Check sheet for the modelled part. Datum: model origin and axes. Units: mm. A direction names the side the tool comes from. Round coordinates to 2 decimals unless told otherwise and drop trailing zeros. Order: outer loops, then holes, each group sorted by start corner. A loop starts at its lowest first (then second) coordinate and runs counter-clockwise, first axis right, second up.
Autodesk Inventor part; units mm, degrees
ref_plane "YZ Plane" through (0, 0, 0) normal (1, 0, 0) x (0, 1, 0)
ref_plane "XZ Plane" through (0, 0, 0) normal (0, 1, 0) x (-1, 0, 0)
ref_plane "XY Plane" through (0, 0, 0) normal (0, 0, 1) x (1, 0, 0)
sketch "Sketch1" plane through (0, 0, 0) normal (0, 0, 1) x (1, 0, 0)
  line L0 (-16.7671, 64.9713) -> (-16.7671, -55.0287)
  line L1 (-16.7671, -55.0287) -> (11.7813, -55.0287)
  line L2 (11.7813, -55.0287) -> (33.2329, -37.0287)
  line L3 (33.2329, -37.0287) -> (33.2329, -21.0287)
  line L4 (33.2329, -21.0287) -> (-16.7671, 64.9713)
  line L5 (-1.7671, -43.0287) -> (-11.7671, -43.0287)
  line L6 (-11.7671, -43.0287) -> (-11.7671, -45.0287)
  line L7 (-11.7671, -45.0287) -> (-1.7671, -45.0287)
  line L8 (-1.7671, -45.0287) -> (-1.7671, -43.0287)
  line L9 (-16.7671, -40.0287) -> (-18.7671, -40.0287)
  line L10 (-18.7671, -40.0287) -> (-18.7671, -10.0287)
  line L11 (-18.7671, -10.0287) -> (-16.7671, -10.0287)
  line L12 (-16.7671, -10.0287) -> (-16.7671, -40.0287)
  line L13 (-16.7671, 9.9713) -> (-18.7671, 9.9713)
  line L14 (-18.7671, 9.9713) -> (-18.7671, 39.9713)
  line L15 (-18.7671, 39.9713) -> (-16.7671, 39.9713)
  line L16 (-16.7671, 39.9713) -> (-16.7671, 9.9713)
  line L17 (-16.7671, 54.9713) -> (-10.9532, 54.9713)
  circle A0 centre (19.2329, -29.0287) radius 9.5
  line L18 (19.2329, -29.0287) -> (33.2329, -29.0287)
  point P0 (0, 0)
  point P1 (-17.7671, -40.0287)
  point P2 (-17.7671, -10.0287)
  dimension "d0" = 120
  dimension "d1" = 10
  dimension "d2" = 2
  dimension "d3" = 10
  dimension "d4" = 5
  dimension "d5" = 2
  dimension "d6" = 30
  dimension "d7" = 15
  dimension "d8" = 2
  dimension "d9" = 30
  dimension "d10" = 20
  dimension "d11" = 18
  dimension "d12" = 16
  dimension "d13" = 50
  dimension "d14" = 10
  dimension "d15" = 50
  dimension "d16" = 19
  dimension "d17" = 36
  dimension "d18" = 90
extrude "Plate1" add sketch "Sketch1" along normal blind 3 contours L17 L4 L3 L2 L1 L0 | L0 L13 L14 L15 | L0 L9 L10 L11
chamfer "Corner Chamfer1" distance 15 angle 45 1 edges at (11.7813, -55.0287, 1.5)
fillet "Corner Round1" radius 17 4 edges at (33.2329, -37.0287, 1.5) (33.2329, -21.0287, 1.5) (23.272, -45.3869, 1.5) (-3.2187, -55.0287, 1.5)
equation "\"d2\" = d19"
equation "\"d5\" = d19"
equation "\"d8\" = d19"
equation "\"d21\" = Thickness"
equation "\"Thickness\" = plate_thickness"
equation "\"BendRadius\" = Thickness"
equation "\"BendReliefWidth\" = Thickness"
equation "\"BendReliefDepth\" = 0.5 * Thickness"
equation "\"CornerReliefSize\" = 4 * Thickness"
equation "\"MinimumRemnant\" = 2 * Thickness"
equation "\"TransitionRadius\" = BendRadius"
equation "\"JacobiRadiusSize\" = BendRadius"
equation "\"GapSize\" = Thickness"
equation "\"A_width\" = 46"
equation "\"A_joint_diameter\" = 16"
equation "\"A_joint_tolerance\" = 3"
equation "\"l___________\" = 0"
equation "\"l__________\" = 0"
equation "\"l_________\" = 0"
equation "\"rivet_diameter\" = 3.35"
equation "\"plate_thickness\" = 3"
equation "\"l________\" = 0"
equation "\"L_Piston_Top\" = 25"
equation "\"L_Piston_Bottom\" = 21"
equation "\"A_B_spacing\" = 2"
equation "\"thin_plate\" = 1.5"
properties part number "Piston_FloorHinge01" material "Stainless Steel"
1) Set-up check for faces 5 (the face through (-12, -55.029, 1)), 6 (the face through (-11.767, -44, 1)), 7 (the face through (-18, -40.029, 1)), 8 (the face through (-16.767, 0, 1)), 9 (the face through (-16.767, 48, 1)): record each of +Z, -Z, +X, -X, +Y, -Y from which the full face is reachable in a straight line by a thin tool's end or side.
2) Sectioned sample at D-D on x = 5.5. Record the cut outline in (y, z), and give its area (3 significant figures).
3) Draft check along Y on faces 1 (the face through (1, -11, 3)), 2 (the face through (-3.31, -54.78, 1.52)), 3 (the face through (-18, 39.971, 1)), 4 (the face through (-18, -10.029, 1)). Enter one of: pulls with the +Y half, pulls with the -Y half, needs draft (parallel to the pull), parting line crosses it, or undercut.
4) Gauge pin test, flat ends, axial feed: pin 1 (0.6 mm diameter, centred on y = -44, z = 2, fed in from -X); pin 2 (1 mm diameter, centred on x = -17.5, z = 1, fed in from +Y); pin 3 (1 mm diameter, centred on x = -18, z = 2, fed in from -Y). Record the tip position at first contact, or that the pin passes through.
5) Sectioned sample at B-B on z = 1.3. Record the cut outline in (x, y), and give its area (3 significant figures).
6) Sectioned sample at A-A on x = 22. Record the cut outline in (y, z), and give its area (3 significant figures).
7) Scan lines: line 1 (Y direction, x = -8, z = 0.8); line 2 (Y direction, x = 17, z = 2.6); line 3 (X direction, y = -23, z = 0.8). Record each from-to range of solid material in increasing order.
8) Sectioned sample at C-C on y = -36. Record the cut outline in (x, z), and give its area (3 significant figures).
Values found:
1. face 5: +Z, -Z, +X, -X, -Y
1. face 6: +Z, -Z
1. face 7: +Z, -Z, -X, -Y
1. face 8: +Z, -Z, -X
1. face 9: +Z, -Z, -X, +Y
2. outline: (-51.86, 0) - (26.67, 0) - (26.67, 3) - (-51.86, 3) - close
2. area: 236 mm2
3. face 1: needs draft
3. face 2: pulls with the -Y half
3. face 3: pulls with the +Y half
3. face 4: undercut
4. pin 1: stops at x = -16.77
4. pin 2: stops at y = 39.97
4. pin 3: stops at y = -40.03
5. outline: (-18.77, -40.03) - (-16.77, -40.03) - (-16.77, -55.03) - (-6.22, -55.03) arc R17 ccw to (-0.4, -54) - (20.46, -46.41) arc R17 ccw to (25.57, -43.46) - (27.16, -42.12) arc R17 ccw to (33.23, -29.1) - (33.23, -25.61) arc R17 ccw to (30.93, -17.07) - (-10.95, 54.97) - (-16.77, 54.97) - (-16.77, 39.97) - (-18.77, 39.97) - (-18.77, 9.97) - (-16.77, 9.97) - (-16.77, -10.03) - (-18.77, -10.03) - close; hole (-11.77, -45.03) - (-1.77, -45.03) - (-1.77, -43.03) - (-11.77, -43.03) - close; hole circle Ø19 at (19.23, -29.03)
5. area: 3,360 mm2
6. outline: (-45.76, 0) - (-38.12, 0) - (-38.12, 3) - (-45.76, 3) - close; (-19.94, 0) - (-1.71, 0) - (-1.71, 3) - (-19.94, 3) - close
6. area: 77.6 mm2
7. line 1: y = -55.03 to -45.03, -43.03 to 49.89
7. line 2: y = -47.67 to -38.26, -19.79 to 6.89
7. line 3: x = -18.77 to 11.89, 26.57 to 33.03
8. outline: (-18.77, 0) - (12.78, 0) - (12.78, 3) - (-18.77, 3) - close; (25.69, 0) - (31.77, 0) - (31.77, 3) - (25.69, 3) - close
8. area: 113 mm2
